Can you work these out from the model? Positions are in its coordinate system, mm. A direction names the side the tool comes from. Give positions to 0.01 mm unless a question says otherwise; leave off trailing zeros. Write each loop counter-clockwise with the first axis right and the second up, starting at its lowest first coordinate (ties: lowest second). Pieces come first, ordered by that corner, then holes. Notation, with made-up numbers: M 58,76.5 L 103,76.5 A14 ccw 103,90.5 Z; hole C 46.5,-39 d8. An arc over 180 degrees is marked long. Write each question's results on one line, items separated by ' | '.
from build123d import *

# Parameters (mm, degrees)
SKETCH_W     = 1000
SKETCH_H     = 1000
PAD_DEPTH    = 1000
SKETCH001_R  = 157.5
PAD001_DEPTH = 1300
SKETCH002_R  = 250
PAD002_DEPTH = 1100


with BuildPart() as part:
    # Sketch → Pad (new body)
    with BuildSketch(Plane.XY):
        Rectangle(SKETCH_W, SKETCH_H)
    extrude(amount=PAD_DEPTH)

    # Sketch001 (on Face6 of Pad) → Pad001 (join)
    with BuildSketch(Plane.XY.offset(1000)):
        Circle(SKETCH001_R)
    extrude(amount=PAD001_DEPTH)

    # Sketch002 (on Face5 of Pad001) → Pad002 (join)
    with BuildSketch(Plane.XY.offset(1000)):
        Circle(SKETCH002_R)
    extrude(amount=PAD002_DEPTH)

    # Sketch003 → Revolution (revolve)
    with BuildSketch(Plane.XZ):
        Polygon((0, 2100), (250, 2100), (157.5, 2400), (0, 2400), align=None)
    revolve(axis=Axis((0, 0, 0), (0, 0, 1)))


solid = part.part
Item 1: I want a section at A-A, the plane x = 0. Please give me the cut outline in (y, z), and give its area (3 significant figures).
Geometry says:
outline: M -500,0 L 500,0 L 500,1000 L 250,1000 L 250,2100 L 157.5,2400 L -157.5,2400 L -250,2100 L -250,1000 L -500,1000 Z | area: 1,670,000 mm2
Item 2: I want a section at D-D, the plane y = -357. Please give me the cut outline in (x, z), and give its area (3 significant figures).
Geometry says:
outline: M -500,0 L 500,0 L 500,1000 L -500,1000 Z | area: 1,000,000 mm2
Item 3: I want a section at C-C, the plane z = 1473. Please give me the cut outline in (x, y), and give its area (3 significant figures).
Geometry says:
outline: C 0,0 d500 | area: 196,000 mm2
Item 4: If I drill on line 1 (Z direction, x = -185, y = -214); line 2 (X direction, y = -119.5, z = 1383.5); line 3 (X direction, y = -148, z = 1674), over which ranges is the centre line in solid material (lowest first)? Write a range as from..to.
Geometry says:
line 1: z = 0..1000 | line 2: x = -219.59..219.59 | line 3: x = -201.48..201.48
Item 5: I'm going to push a flat-ended pin straight in: pin 1 (12 mm diameter, centred on x = 299.5, y = 58.5, fed in from +Z). Where does the tip first touch, or does it pass through?
Geometry says:
pin 1: stops at z = 1000
Item 6: For faces 1 (the face through (-7, -500, 493)), 2 (the face through (-249.76, 10.99, 1542.3)), which set-ups out of +Z, -Z, +X, -X, +Y, -Y let a thin tool reach every point of the face, with its end or its side?
Geometry says:
face 1: +Z, -Z, +X, -X, -Y | face 2: +Z
